from build123d import *

# Parameters (mm, degrees)
BOSS_EXTRUDE1_START = -40.2844
BOSS_EXTRUDE1_DEPTH = 40.2844
SKETCH2_R           = 2.1336
CUT_EXTRUDE1_DEPTH  = 72.997408865
SKETCH3_R           = 3.9878
CUT_EXTRUDE2_DEPTH  = 4
SKETCH4_R           = 2.5
CUT_EXTRUDE3_DEPTH  = 138.863130216


# Read off the part's stored shape, not the designer's step: Boss-Extrude1
with BuildPart() as part:
    # Boss-Extrude1 outline → Boss-Extrude1 (new body)
    with BuildSketch(Plane.XY.offset(BOSS_EXTRUDE1_START)):
        with BuildLine():
            ThreePointArc((15.75, 111.352890045), (18.130636083, 117.100253962), (23.878, 119.480890045))
            Line((23.878, 119.480890045), (55.12, 119.480890045))
            Line((55.12, 119.480890045), (55.12, 125.830890045))
            Line((55.12, 125.830890045), (9.4, 125.830890045))
            Line((9.4, 125.830890045), (9.4, 96.620890045))
            Line((9.4, 96.620890045), (15.75, 96.620890045))
            Line((15.75, 96.620890045), (15.75, 111.352890045))
        make_face()
    extrude(amount=BOSS_EXTRUDE1_DEPTH)

    # Sketch2 → Cut-Extrude1 (cut, through all)
    with BuildSketch(Plane(origin=(0, 119.480890045, 0), x_dir=(-1, 0, 0), z_dir=(0, -1, 0))):
        with Locations(Location((-47.756789836, 13.03483709, 0), (0, 0, 90))):
            Circle(SKETCH2_R)
        with Locations(Location((-34.133741301, 26.657885626, 0), (0, 0, 90))):
            Circle(SKETCH2_R)
    extrude(amount=-CUT_EXTRUDE1_DEPTH, mode=Mode.SUBTRACT)

    # Sketch3 → Cut-Extrude2 (cut)
    with BuildSketch(Plane(origin=(0, 125.830890045, 0), x_dir=(1, 0, 0), z_dir=(0, 1, 0))):
        with Locations(Location((47.756789836, 13.03483709, 0), (0, 0, 270))):
            Circle(SKETCH3_R)
        with Locations(Location((34.133741301, 26.657885626, 0), (0, 0, 270))):
            Circle(SKETCH3_R)
    extrude(amount=-CUT_EXTRUDE2_DEPTH, mode=Mode.SUBTRACT)

    # Sketch4 → Cut-Extrude3 (cut, through all)
    with BuildSketch(Plane(origin=(15.75, 0, 0), x_dir=(0, 0, -1), z_dir=(1, 0, 0))):
        with Locations((10.0711, 103.986890045)):
            Circle(SKETCH4_R)
        with Locations((30.2133, 103.986890045)):
            Circle(SKETCH4_R)
    extrude(amount=-CUT_EXTRUDE3_DEPTH, mode=Mode.SUBTRACT)


solid = part.part
Work out the finished part from the listing and answer in its coordinate system (mm). A direction names the side the tool comes from. Give positions to 0.01 mm unless a question says otherwise; leave off trailing zeros. Loops run counter-clockwise (first coordinate to the right, second up) from the corner with the lowest first, then second, coordinate; pieces in that order, holes last. Notation, with made-up numbers: M 67.25,56 L 96.25,56 A37 cw 96.25,93 Z; hole C 15,79 d9. An arc over 180 degrees is marked long. Use CSV: the item, a comma, the result in double quotes.
1) Determine the mould class of faces 4 (the flat face through (55.12, 123, -20)), 5 (the flat face through (32, 121.831, -25)), 6 (the flat face through (9.4, 111, -20)), 7 (the flat face through (33, 125.831, -20)) for opening direction X: released by +X, released by -X, zero draft, split by the parting line, or undercut.
Answer:
face 4,"released by +X"
face 5,"undercut"
face 6,"released by -X"
face 7,"zero draft"
2) Consider L1, parallel to Y at x = 52, z = -2; L2, parallel to X at y = 99.75, z = -36; L3, parallel to Y at x = 12.5, z = -8. Determine where each line is inside the solid, lowest interval first.
Answer:
L1,"119.48 to 125.83"
L2,"9.4 to 15.75"
L3,"96.62 to 102.59, 105.39 to 125.83"
3) Given P1, Ø7, axis at x = 34.13, z = -26.66, coming from the +Y side; P2, Ø10, axis at x = 26, z = -17, coming from the -Y side; P3, Ø6.5, axis at x = 47.76, z = -13.03, coming from the -Y side, each flat-ended and moving along its own axis, determine where each tip first touches the part or whether it passes through.
Answer:
P1,"y = 121.83"
P2,"y = 118.95"
P3,"y = 119.48"
4) Find section D-D on y = 123.5. Write down the section's boundary in (x, z).
Answer:
outline,"M 9.4,-40.28 L 55.12,-40.28 L 55.12,0 L 9.4,0 Z; hole C 34.13,-26.66 d7.98; hole C 47.76,-13.03 d7.98"
5) Find section B-B on x = 13. Write down the section's boundary in (y, z).
Answer:
outline,"M 96.62,-40.28 L 125.83,-40.28 L 125.83,0 L 96.62,0 Z; hole C 103.99,-30.21 d5; hole C 103.99,-10.07 d5"
6) Find section C-C on x = 26.5. Write down the section's boundary in (y, z), plus the area to 3 significant figures.
Answer:
outline,"M 119.48,-40.28 L 125.83,-40.28 L 125.83,0 L 119.48,0 Z"
area,"256 mm^2"
7) Find section A-A on z = -2.5. Write down the section's boundary in (x, y), plus the area to 3 significant figures.
Answer:
outline,"M 9.4,96.62 L 15.75,96.62 L 15.75,111.35 A8.13 cw 23.88,119.48 L 55.12,119.48 L 55.12,125.83 L 9.4,125.83 Z"
area,"450 mm^2"
8) Which of the six approach directions +Z, -Z, +X, -X, +Y, -Y give full straight-line access (tool end or side, diameter ignored) to faces 1 (the cylindrical face through (30.24, 123.86, -27.52)), 2 (the cylindrical face through (35.933, 120.639, -27.805)), 3 (the flat face through (15.75, 104, -20))?
Answer:
face 1,"+Y"
face 2,"+Y, -Y"
face 3,"+Z, -Z, +X, -Y"
